from build123d import *

# Parameters (mm, degrees)
SKETCH1_R                     = 6.35
MAIN_BODY_BOSS_EXTRUDE1_DEPTH = 66.04
SKETCH2_R                     = 3.175
TENDON_1_BOSS_EXTRUDE2_DEPTH  = 6.096
TENDON_START                  = 6.096
SKETCH3_R                     = 3.175
TENDON_2_BOSS_EXTRUDE3_DEPTH  = 6.096
SKETCH4_R                     = 1.7526
F_10_32_CUT_EXTRUDE1_DEPTH    = 11.176
F_10_32_START                 = -11.176
SKETCH5_R                     = 1.7526
F_10_32_CUT_EXTRUDE2_DEPTH    = 11.176
CHAMFER1_SIZE                 = 0.381
CUT_EXTRUDE3_DEPTH            = 73.692829743
CUT_EXTRUDE3_DEPTH_BACK       = 73.692829743
SKETCH6_R                     = 3.175


with BuildPart() as part:
    # Sketch1 → Main Body Boss-Extrude1 (new body)
    with BuildSketch(Plane(origin=(0, 0, 0), x_dir=(1, 0, 0), z_dir=(0, 1, 0))):
        with Locations(Location((0, 0, 0), (0, 0, 270))):
            Circle(SKETCH1_R)
    extrude(amount=MAIN_BODY_BOSS_EXTRUDE1_DEPTH)

    # Sketch2 → Tendon 1 Boss-Extrude2 (add)
    with BuildSketch(Plane.XZ):
        with Locations(Location((0, 0, 0), (0, 0, 90))):
            Circle(SKETCH2_R)
    extrude(amount=TENDON_1_BOSS_EXTRUDE2_DEPTH)

    # Sketch3 → Tendon 2 Boss-Extrude3 (add)
    with BuildSketch(Plane(origin=(0, 66.04, 0), x_dir=(1, 0, 0), z_dir=(0, 1, 0)).offset(TENDON_START)):
        with Locations(Location((0, 0, 0), (0, 0, 270))):
            Circle(SKETCH3_R)
    extrude(amount=-TENDON_2_BOSS_EXTRUDE3_DEPTH)

    # Sketch4 → 10_32 Cut-Extrude1 (cut)
    with BuildSketch(Plane(origin=(0, 72.136, 0), x_dir=(1, 0, 0), z_dir=(0, 1, 0))):
        with Locations(Location((0, 0, 0), (0, 0, 270))):
            Circle(SKETCH4_R)
    extrude(amount=-F_10_32_CUT_EXTRUDE1_DEPTH, mode=Mode.SUBTRACT)

    # Sketch5 → 10_32 Cut-Extrude2 (cut)
    with BuildSketch(Plane.XZ.offset(6.096).offset(F_10_32_START)):
        with Locations(Location((0, 0, 0), (0, 0, 90))):
            Circle(SKETCH5_R)
    extrude(amount=F_10_32_CUT_EXTRUDE2_DEPTH, mode=Mode.SUBTRACT)

    # Chamfer1
    chamfer1_edges = [part.edges().sort_by_distance(p)[0] for p in [
        (0, 72.136, -3.175),
        (0, 0, -6.35),
        (0, 66.04, -6.35),
        (0, -6.096, -3.175),
    ]]
    chamfer(chamfer1_edges, length=CHAMFER1_SIZE)

    # Sketch6 → Cut-Extrude3 (cut, two sides: drawn at the far end of the back side and taken through both)
    with BuildSketch(Plane(origin=(0, 0, 0), x_dir=(0, 0, -1), z_dir=(1, 0, 0)).offset(-CUT_EXTRUDE3_DEPTH_BACK)):
        with Locations((0, 32.8295)):
            Circle(SKETCH6_R)
    extrude(amount=CUT_EXTRUDE3_DEPTH + CUT_EXTRUDE3_DEPTH_BACK, mode=Mode.SUBTRACT)


solid = part.part
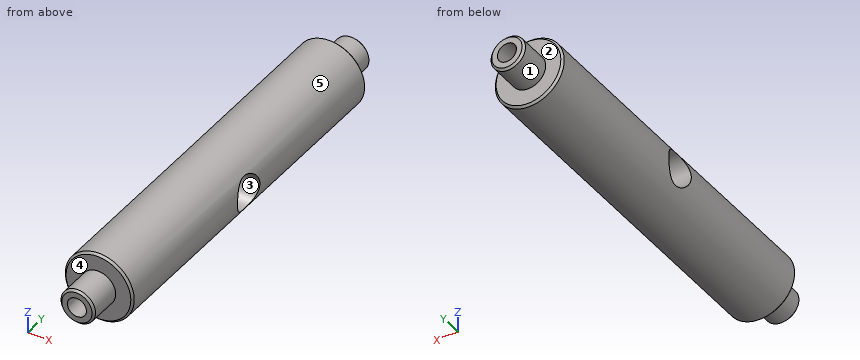
The model under review builds one solid part; all positions refer to its coordinate system, in mm. Face numbers are marked on the shaded views. A direction names the side the tool comes from. Coordinates: 2 decimals unless noted, no trailing zeros. Loops run counter-clockwise (first coordinate to the right, second up) from the corner with the lowest first, then second, coordinate; pieces in that order, holes last. Notation, with made-up numbers: (-36.5, -20.5) -> (15.5, -20.5) arc R35 ccw to (15.5, 17.5) -> close; hole circle Ø9 at (-28.5, 36). An arc over 180 degrees is marked (long way). Use a Markdown table: item, result. Add a question column.
1. Draft analysis for pull direction Y (two halves, no side actions). For the marked faces 1, 2 and 3, state which applies: pulls with the +Y half, pulls with the -Y half, needs draft (parallel to the pull), parting line crosses it, or undercut.
2. Clearance check with flat-ended pins moving along their axes: pin 1 Ø1.1 at (x, z) = (-0.5, 1) entering from +Y; pin 2 Ø1.1 at (x, z) = (0.5, -0.5) entering from -Y. State where each tip first meets the part, or that it passes through.
3. Add section C-C on y = 40. Write out the cut boundary in (x, z), plus the area to 3 significant figures.
4. Machinability: for the marked faces 4 and 5, which of the approach directions +Z, -Z, +X, -X, +Y, -Y give a long, thin tool a straight path to every point of the face, cutting with its end or side? Answer none if there is none.
5. To check wall thickness, follow line 1 (Y direction, x = -2, z = 0); line 2 (Y direction, x = -0.5, z = 0); line 3 (X direction, y = -0.5, z = 0) (3 decimals). State the ranges of each line that lie inside material, in increasing order.
Returned:
| question | item | result |
|---|---|---|
| 1 | face 1 | needs draft |
| 1 | face 2 | pulls with the +Y half |
| 1 | face 3 | undercut |
| 2 | pin 1 | stops at y = 60.96 |
| 2 | pin 2 | stops at y = 5.08 |
| 3 | outline | circle Ø12.7 at (0, 0) |
| 3 | area | 127 mm² |
| 4 | face 4 | -Y |
| 4 | face 5 | +Y, -Y |
| 5 | line 1 | y = -6.1 to 29.65, 36 to 72.14 |
| 5 | line 2 | y = 5.08 to 29.65, 36 to 60.96 |
| 5 | line 3 | x = -3.175 to -1.753, 1.753 to 3.175 |
